The model under review builds one solid part; all positions refer to its coordinate system, in mm. A direction names the side the tool comes from. Give positions to 0.01 mm unless a question says otherwise; leave off trailing zeros. Loops run counter-clockwise (first coordinate to the right, second up) from the corner with the lowest first, then second, coordinate; pieces in that order, holes last. Notation, with made-up numbers: (6.5, 37) - (25.5, 37) arc R26 cw to (25.5, 75) - close; hole circle Ø8 at (9.5, 86). An arc over 180 degrees is marked (long way). Answer as a JSON object with one key per item and string values.
from build123d import *

# Parameters (mm, degrees)
SKETCH1_W           = 16
SKETCH1_H           = 90
BOSS_EXTRUDE1_DEPTH = 2
SKETCH2_W           = 1.5
SKETCH2_H           = 90
BOSS_EXTRUDE2_DEPTH = 4
SKETCH3_W           = 1.5
SKETCH3_H           = 90
BOSS_EXTRUDE3_DEPTH = 1.5
SKETCH4_W           = 1.5
SKETCH4_H           = 90
BOSS_EXTRUDE4_DEPTH = 1.5
SKETCH6_W           = 6
SKETCH6_H           = 90
BOSS_EXTRUDE5_DEPTH = 7
SKETCH7_W           = 6
SKETCH7_H           = 90
BOSS_EXTRUDE6_DEPTH = 7


with BuildPart() as part:
    # Sketch1 → Boss-Extrude1 (new body)
    with BuildSketch(Plane.XY):
        with Locations((0, -20)):
            Rectangle(SKETCH1_W, SKETCH1_H)
    extrude(amount=BOSS_EXTRUDE1_DEPTH)

    # Sketch2 → Boss-Extrude2 (add)
    with BuildSketch(Plane.XY.offset(2)):
        with Locations((-7.25, -20)):
            Rectangle(SKETCH2_W, SKETCH2_H)
        with Locations((7.25, -20)):
            Rectangle(SKETCH2_W, SKETCH2_H)
    extrude(amount=BOSS_EXTRUDE2_DEPTH)

    # Sketch3 → Boss-Extrude3 (add)
    with BuildSketch(Plane(origin=(-6.5, 0, 0), x_dir=(0, 0, -1), z_dir=(1, 0, 0))):
        with Locations((-5.25, -20)):
            Rectangle(SKETCH3_W, SKETCH3_H)
    extrude(amount=BOSS_EXTRUDE3_DEPTH)

    # Sketch4 → Boss-Extrude4 (add)
    with BuildSketch(Plane.ZY.offset(-6.5)):
        with Locations((5.25, -20)):
            Rectangle(SKETCH4_W, SKETCH4_H)
    extrude(amount=BOSS_EXTRUDE4_DEPTH)

    # Sketch6 → Boss-Extrude5 (add)
    with BuildSketch(Plane(origin=(8, 0, 0), x_dir=(0, 0, -1), z_dir=(1, 0, 0))):
        with Locations((-3, -20)):
            Rectangle(SKETCH6_W, SKETCH6_H)
    extrude(amount=BOSS_EXTRUDE5_DEPTH)

    # Sketch7 → Boss-Extrude6 (add)
    with BuildSketch(Plane.ZY.offset(8)):
        with Locations((3, -20)):
            Rectangle(SKETCH7_W, SKETCH7_H)
    extrude(amount=BOSS_EXTRUDE6_DEPTH)


solid = part.part
Q1. For faces 1 (the face through (6, -21, 4.5)), 2 (the face through (-5, -19, 5)), 3 (the face through (0.2, 25, 1.6)), list the 3-axis set-ups (+Z, -Z, +X, -X, +Y, -Y) from which the entire face can be reached by the end or side of a thin tool; tool diameter is ignored.
Results:
{"face 1": "+Y, -Y", "face 2": "+Z, +Y, -Y", "face 3": "+Z, -Z, +X, -X, +Y"}
Q2. Consider section B-B, the plane y = -56. State the section outline as (x, z) points.
Results:
{"outline": "(-15, 0) - (15, 0) - (15, 6) - (5, 6) - (5, 4.5) - (6.5, 4.5) - (6.5, 2) - (-6.5, 2) - (-6.5, 4.5) - (-5, 4.5) - (-5, 6) - (-15, 6) - close"}
Q3. The part is to be moulded in two halves that separate along X. For faces 4 (the face through (6.5, -21, 3)), 5 (the face through (-6, -21, 4.5)), 6 (the face through (-10, -21, 6)), 7 (the face through (-15, -19, 3)), say which applies: +X half, -X half, draft (parallel to the pull), parting line (faces both ways), or undercut.
Results:
{"face 4": "undercut", "face 5": "undercut", "face 6": "draft", "face 7": "-X half"}
Q4. Consider section A-A, the plane z = 3.5. State the section outline as (x, y) points, plus the area to 3 significant figures.
Results:
{"outline": "(-15, -65) - (-6.5, -65) - (-6.5, 25) - (-15, 25) - close; (6.5, -65) - (15, -65) - (15, 25) - (6.5, 25) - close", "area": "1,530 mm^2"}
Q5. Consider section C-C, the plane x = -3. State the section outline as (y, z) points, plus the area to 3 significant figures.
Results:
{"outline": "(-65, 0) - (25, 0) - (25, 2) - (-65, 2) - close", "area": "180 mm^2"}
Q6. To check wall thickness, follow probe 1 along X at (y, z) = (-60, 3.05); probe 2 along X at (y, z) = (-5.5, 4.6); probe 3 along Z at (x, y) = (-1.5, -10.5). State the ranges of each line that lie inside material, in increasing order. Write a range as [from, to].
Results:
{"probe 1": "x = [-15, -6.5], [6.5, 15]", "probe 2": "x = [-15, -5], [5, 15]", "probe 3": "z = [0, 2]"}
